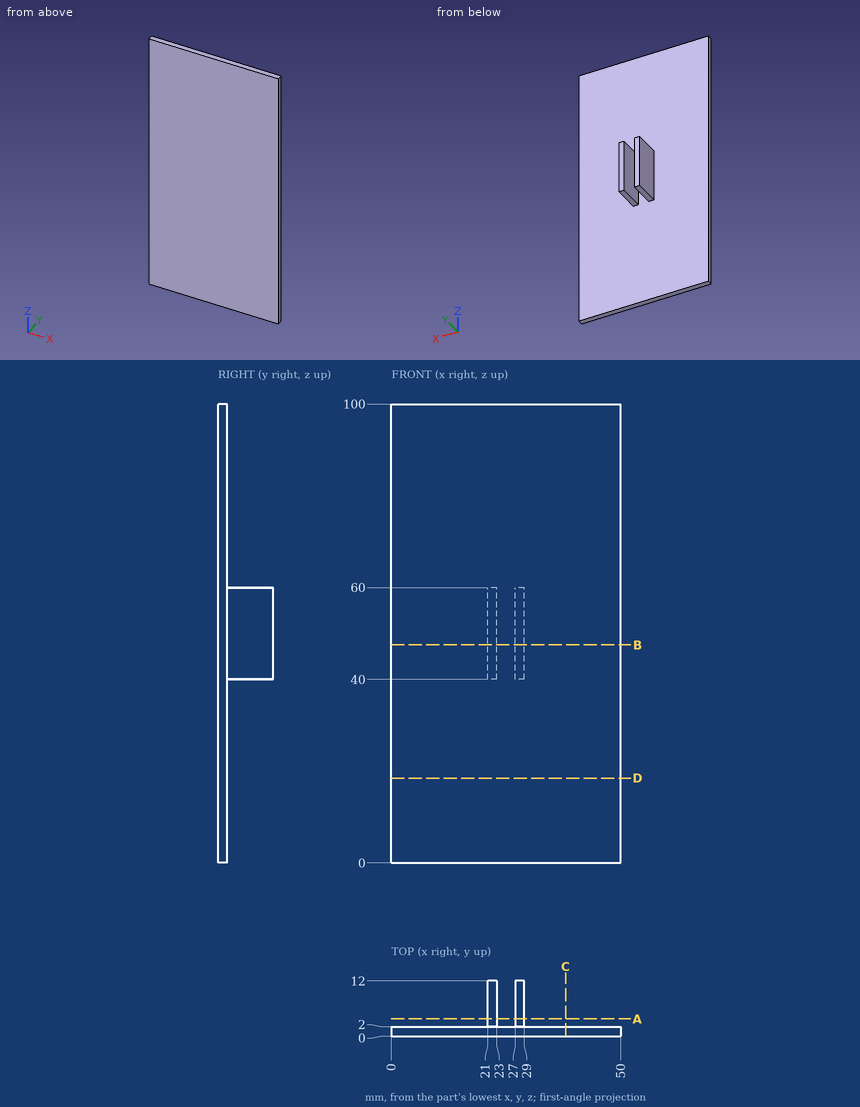
Could you check a few things on this drawing? It's one solid part, dimensions in mm from its lowest x, y, z. Give positions to 0.01 mm unless a question says otherwise; leave off trailing zeros. Write each loop counter-clockwise with the first axis right and the second up, starting at its lowest first coordinate (ties: lowest second). Pieces come first, ordered by that corner, then holes. Notation, with made-up numbers: (85.5, 59.5) - (94.5, 59.5) arc R23 cw to (94.5, 73.5) - close; hole circle Ø9 at (-21.5, -0.75). An arc over 180 degrees is marked (long way). Use CSV: the item, a comma, the result in double quotes. Start each with the question number.
Item 1: If I drill on line 1 along X through (y, z) = (7, 48.5); line 2 along Y through (x, z) = (27, 61); line 3 along Z through (x, y) = (28, 3), over which ranges is the centre line in solid material (lowest first)?
Item 2: I want a section at B-B, the plane z = 47.5. Please give me the cut outline in (x, y).
Item 3: I want a section at A-A, the plane y = 3.75. Please give me the cut outline in (x, z).
Item 4: I want a section at C-C, the plane x = 38. Please give me the cut outline in (y, z), then the cut area to 3 significant figures.
Item 5: I'm going to push flat-ended pins straight in: pin 1 (12 mm diameter, centred on x = 37.5, z = 13, fed in from -Y); pin 2 (3 mm diameter, centred on y = 8.5, z = 54, fed in from +X); pin 3 (1.6 mm diameter, centred on x = 27.5, y = 6.5, fed in from +Z); pin 4 (1 mm diameter, centred on x = 37, z = 46, fed in from +Y). Where does each tip first touch, or does it pass through?
Item 6: I want a section at D-D, the plane z = 18.5. Please give me the cut outline in (x, y), then the cut area to 3 significant figures.
Findings:
1,line 1,"x = 21 to 23, 27 to 29"
1,line 2,"y = 0 to 2"
1,line 3,"z = 40 to 60"
2,outline,"(0, 0) - (50, 0) - (50, 2) - (29, 2) - (29, 12) - (27, 12) - (27, 2) - (23, 2) - (23, 12) - (21, 12) - (21, 2) - (0, 2) - close"
3,outline,"(21, 40) - (23, 40) - (23, 60) - (21, 60) - close; (27, 40) - (29, 40) - (29, 60) - (27, 60) - close"
4,outline,"(0, 0) - (2, 0) - (2, 100) - (0, 100) - close"
4,area,"200 mm2"
5,pin 1,"stops at y = 0"
5,pin 2,"stops at x = 29"
5,pin 3,"stops at z = 60"
5,pin 4,"stops at y = 2"
6,outline,"(0, 0) - (50, 0) - (50, 2) - (0, 2) - close"
6,area,"100 mm2"
